```python
from build123d import *

# Parameters (mm, degrees)
F1_DEPTH = 100
F2_W     = 46
F2_H     = 96
F3_DEPTH = 15
F4_R     = 8.5
F5_DEPTH = 50.2
F6_R     = 8.5
F7_DEPTH = 63.4


with BuildPart() as f1:
    # F0 (on Front) → F1 (new body)
    with BuildSketch(Plane.XZ):
        Polygon((-25, -8.442136), (0, -8.442136), (25, -8.442136), (25, 6.557864), (39.142136, 20.7), (21.464466, 38.377669), (7.32233, 24.235533), (0, 24.235533), (-7.32233, 24.235533), (-21.464466, 38.377669), (-39.142136, 20.7), (-25, 6.557864), align=None)
    extrude(amount=F1_DEPTH)

    # F2 (on face) → F3 (cut)
    with BuildSketch(Plane(origin=(0, 0, -8.442136), x_dir=(1, 0, 0), z_dir=(0, 0, -1))):
        with Locations((0, 50)):
            Rectangle(F2_W, F2_H)
    extrude(amount=-F3_DEPTH, mode=Mode.SUBTRACT)

    # F4 (on face) → F5 (cut)
    with BuildSketch(Plane(origin=(29.921068, 0, 29.921068), x_dir=(0.707107, 0, -0.707107), z_dir=(0.707107, 0, 0.707107))):
        with Locations((-0.046836, -87.5)):
            Circle(F4_R)
        with Locations((0.54056, -62.5)):
            Circle(F4_R)
        with Locations((0.54056, -37.5)):
            Circle(F4_R)
        with Locations((0.54056, -12.5)):
            Circle(F4_R)
    extrude(amount=-F5_DEPTH, mode=Mode.SUBTRACT)

    # F6 (on face) → F7 (cut)
    with BuildSketch(Plane(origin=(-29.921068, 0, 29.921068), x_dir=(0.707107, 0, 0.707107), z_dir=(-0.707107, 0, 0.707107))):
        with Locations((-0.54056, -12.5)):
            Circle(F6_R)
        with Locations((-0.54056, -37.5)):
            Circle(F6_R)
        with Locations((-0.54056, -62.5)):
            Circle(F6_R)
        with Locations((-0.54056, -87.5)):
            Circle(F6_R)
    extrude(amount=-F7_DEPTH, mode=Mode.SUBTRACT)


solid = f1.part
```
The model under review builds one solid part; all positions refer to its coordinate system, in mm. A direction names the side the tool comes from. Round coordinates to 2 decimals unless told otherwise and drop trailing zeros. Loops run counter-clockwise (first coordinate to the right, second up) from the corner with the lowest first, then second, coordinate; pieces in that order, holes last. Notation, with made-up numbers: (-12.5, 74) -> (46.5, 74) arc R16 ccw to (46.5, 98) -> close; hole circle Ø6 at (62.25, -27.75). An arc over 180 degrees is marked (long way). Answer as a JSON object with one key per item and string values. Group by question number.
1) We need section A-A on y = -58.5. Write out the cut boundary in (x, z), then the cut area to 3 significant figures.
2) We need section C-C on y = -76. Write out the cut boundary in (x, z).
3) We need section D-D on z = 22. Give the number of separate pieces and of enclosed holes in the cut face, then the cut area to 3 significant figures.
4) For line 1 (X direction, y = -41.5, z = 1); line 2 (Y direction, x = -20, z = 18); line 3 (X direction, y = -92, z = 21), list the stretches that pass through material, from the lowest coordinate up. Write a range as [from, to].
5) For faces 4 (the face through (0, -98, -1)), 5 (the face through (-30.18, -49.3, 29.66)), 6 (the face through (-25, -49, -1)), 7 (the face through (25, -49, -1)), 8 (the face through (0, -49, 24.236)), list the 3-axis set-ups (+Z, -Z, +X, -X, +Y, -Y) from which the entire face can be reached by the end or side of a thin tool; tool diameter is ignored.
6) For pin 1 Ø1.5 at (y, z) = (-15.5, 18.5) entering from +X; pin 2 Ø5 at (y, z) = (-48.5, 24) entering from +X; pin 3 Ø12 at (y, z) = (-39.5, 1.5) entering from +X, all flat-tipped, find the tip position at first contact; note any pin that passes through.
7) We need section B-B on z = 4.5. Write out the cut boundary in (x, y), then the cut area to 3 significant figures.
8) Mouldability with a two-part tool opening along Z and no side actions: class faces 1 (the face through (0, -2, -1)), 2 (the face through (14.124, -62.126, 25.369)), 3 (the face through (0, -51, 6.558)) as released by +Z, released by -Z, zero draft, split by the parting line, or undercut.
Result set:
{
 "1": {"outline": "(-39.14, 20.7) -> (-25, 6.56) -> (-25, -8.44) -> (-23, -8.44) -> (-23, 6.56) -> (-17.93, 6.56) -> (-35.61, 24.24) -> close; (-25, 34.84) -> (0, 9.84) -> (25, 34.84) -> (21.46, 38.38) -> (7.32, 24.24) -> (-7.32, 24.24) -> (-21.46, 38.38) -> close; (17.93, 6.56) -> (23, 6.56) -> (23, -8.44) -> (25, -8.44) -> (25, 6.56) -> (39.14, 20.7) -> (35.61, 24.24) -> close", "area": "667 mm²"},
 "2": {"outline": "(-39.14, 20.7) -> (-25, 6.56) -> (-25, -8.44) -> (-23, -8.44) -> (-23, 6.56) -> (23, 6.56) -> (23, -8.44) -> (25, -8.44) -> (25, 6.56) -> (39.14, 20.7) -> (21.46, 38.38) -> (7.32, 24.24) -> (-7.32, 24.24) -> (-21.46, 38.38) -> close"},
 "3": {"separate pieces": "1", "enclosed holes": "8", "area": "5,000 mm²"},
 "4": {"line 1": "[-25, -23], [23, 25]", "line 2": "[-100, -95.95], [-79.05, -70.95], [-54.05, -45.95], [-29.05, -20.95], [-4.05, 0]", "line 3": "[-38.84, -31.96], [-11.57, 10.74], [31.13, 38.84]"},
 "5": {"face 4": "-Z", "face 5": "+Z, -X, +Y, -Y", "face 6": "-Z, -X, +Y, -Y", "face 7": "-Z, +X, +Y, -Y", "face 8": "+Z, +Y, -Y"},
 "6": {"pin 1": "x = 37.69", "pin 2": "x = 38.34", "pin 3": "x = 25.94"},
 "7": {"outline": "(-25, -100) -> (25, -100) -> (25, 0) -> (-25, 0) -> close; hole (-23, -98) -> (23, -98) -> (23, -2) -> (-23, -2) -> close", "area": "584 mm²"},
 "8": {"face 1": "zero draft", "face 2": "undercut", "face 3": "released by -Z"}
}
